Could you check a few things on this drawing? It's one solid part, dimensions in mm from its lowest x, y, z. Coordinates: 2 decimals unless noted, no trailing zeros. Write each loop counter-clockwise with the first axis right and the second up, starting at its lowest first coordinate (ties: lowest second). Pieces come first, ordered by that corner, then holes. Notation, with made-up numbers: (-25.75, -20) - (-19.75, -20) arc R28 ccw to (-19.75, 19) - close; hole circle Ø2 at (69.25, 80). An arc over 180 degrees is marked (long way). Answer as a JSON object with one key per item and string values. Group by question number.
1) If we section it at A-A (x = 1.3): State how many separate pieces and enclosed holes the cut face has, plus the area to 3 significant figures.
2) Please list where these lines run through material, in increasing order: line 1 along Y through (x, z) = (1.9, 62); line 2 along X through (y, z) = (3.25, 76.5); line 3 along Y through (x, z) = (3.35, 77.5).
3) If we section it at B-B (z = 54): Write out the boundary of the cut face in (x, y), plus the area to 3 significant figures.
4) Will these pins go through, and if not, where does the flat tip stop? pin 1 Ø5.5 at (y, z) = (6, 38) entering from +X; pin 2 Ø1 at (x, y) = (2, 7.5) entering from +Z; pin 3 Ø2 at (x, y) = (3.5, 9) entering from -Z.
5) We'd pull the mould along Y, two halves only. Please class the marked faces 1 and 2: released by +Y, released by -Y, zero draft, split by the parting line, or undercut.
6) If we section it at C-C (z = 75): Write out the boundary of the cut face in (x, y).
7) If we section it at D-D (y = 1): Write out the boundary of the cut face in (x, z).
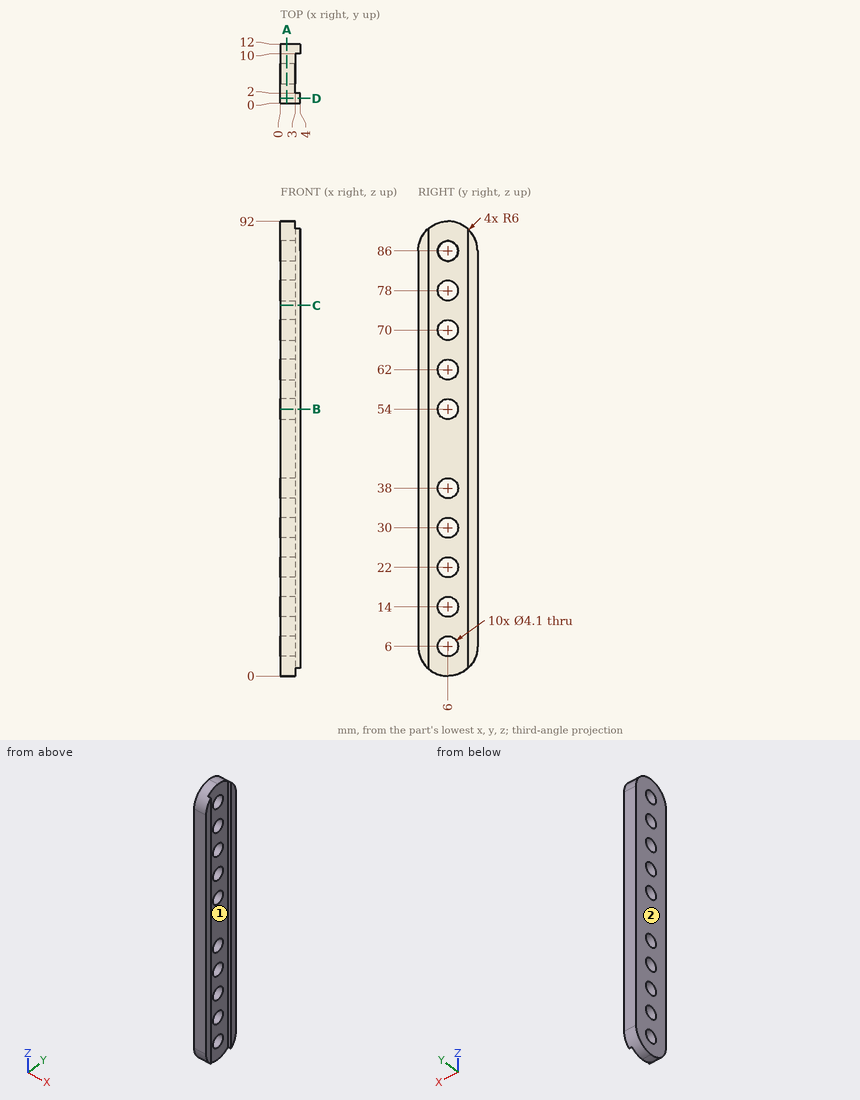
Here are the results:
{
 "1": {"separate pieces": "1", "enclosed holes": "10", "area": "941 mm²"},
 "2": {"line 1": "y = 0 to 3.95, 8.05 to 12", "line 2": "x = 0 to 3", "line 3": "y = 0 to 2, 10 to 12"},
 "3": {"outline": "(0, 0) - (4, 0) - (4, 2) - (3, 2) - (3, 3.95) - (0, 3.95) - close; (0, 8.05) - (3, 8.05) - (3, 10) - (4, 10) - (4, 12) - (0, 12) - close", "area": "27.7 mm²"},
 "4": {"pin 1": "stops at x = 3", "pin 2": "stops at z = 91.92", "pin 3": "stops at z = 0.39"},
 "5": {"face 1": "undercut", "face 2": "zero draft"},
 "6": {"outline": "(0, 0) - (4, 0) - (4, 2) - (3, 2) - (3, 10) - (4, 10) - (4, 12) - (0, 12) - close"},
 "7": {"outline": "(0, 2.68) - (4, 2.68) - (4, 89.32) - (0, 89.32) - close"}
}
